Can you work these out from the model? Positions are in its coordinate system, mm. Face numbers are marked on the shaded views. A direction names the side the tool comes from. Give positions to 0.01 mm unless a question says otherwise; leave off trailing zeros. Write each loop counter-clockwise with the first axis right and the second up, starting at its lowest first coordinate (ties: lowest second). Pieces come first, ordered by that corner, then holes. Notation, with made-up numbers: (70.25, 42) -> (93.25, 42) arc R22 cw to (93.25, 62) -> close; hole circle Ø2 at (69, -35). An arc over 180 degrees is marked (long way). One line per item, written item: value.
from build123d import *

# Parameters (mm, degrees)
SKETCH1_R               = 1.5
BOSS_EXTRUDE1_DEPTH     = 1.5
SKETCH5_W               = 7.463090523
SKETCH5_H               = 8
BOSS_EXTRUDE2_DEPTH     = 3.5
CUT_EXTRUDE1_DEPTH      = 7
CUT_EXTRUDE1_DEPTH_BACK = 6
SKETCH2_W               = 2.5
SKETCH2_H               = 5.25
SKETCH3_R               = 2
CUT_EXTRUDE2_DEPTH      = 3
SKETCH6_W               = 5
SKETCH6_H               = 4
CUT_EXTRUDE3_DEPTH      = 3.5


with BuildPart() as part:
    # Sketch1 → Boss-Extrude1 (new, symmetric)
    with BuildSketch(Plane.XY):
        with BuildLine():
            Line((12, 4), (0, 4))
            ThreePointArc((0, 4), (-4, 0), (0, -4))
            Line((0, -4), (12, -4))
            Line((12, -4), (12, 4))
        make_face()
        Circle(SKETCH1_R, mode=Mode.SUBTRACT)
    extrude(amount=BOSS_EXTRUDE1_DEPTH, both=True)

    # Sketch5 → Boss-Extrude2 (add, symmetric)
    with BuildSketch(Plane.XY):
        with Locations((8.268454739, 0)):
            Rectangle(SKETCH5_W, SKETCH5_H)
    extrude(amount=BOSS_EXTRUDE2_DEPTH, both=True)

    # Sketch2 → Cut-Extrude1 (cut, two sides: drawn at the far end of the back side and taken through both)
    with BuildSketch(Plane.XY.offset(1.5).offset(-CUT_EXTRUDE1_DEPTH_BACK)):
        with Locations((8.25, 0)):
            Rectangle(SKETCH2_W, SKETCH2_H)
    extrude(amount=CUT_EXTRUDE1_DEPTH + CUT_EXTRUDE1_DEPTH_BACK, mode=Mode.SUBTRACT)

    # Sketch3 → Cut-Extrude2 (cut)
    with BuildSketch(Plane(origin=(12, 0, 0), x_dir=(0, 0, -1), z_dir=(1, 0, 0))):
        with Locations(Location((0, 0, 0), (0, 0, 90))):
            Circle(SKETCH3_R)
    extrude(amount=-CUT_EXTRUDE2_DEPTH, mode=Mode.SUBTRACT)

    # Sketch6 → Cut-Extrude3 (cut)
    with BuildSketch(Plane(origin=(0, 0, -3.5), x_dir=(-1, 0, 0), z_dir=(0, 0, -1))):
        with Locations((-12, 0)):
            Rectangle(SKETCH6_W, SKETCH6_H)
    extrude(amount=-CUT_EXTRUDE3_DEPTH, mode=Mode.SUBTRACT)


solid = part.part
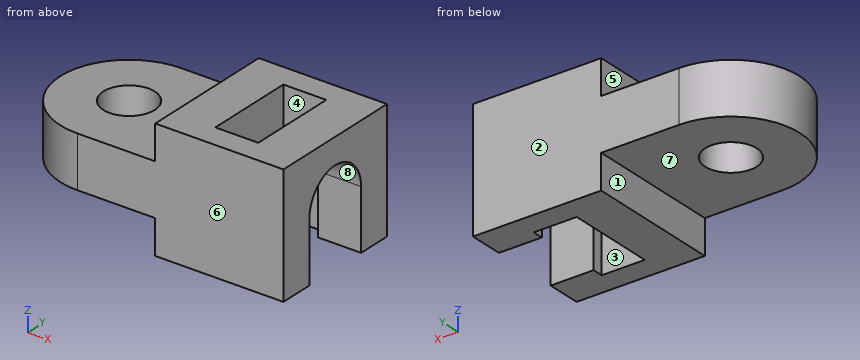
1) If we section it at C-C (x = -0.25): Write out the boundary of the cut face in (y, z).
Answer list:
outline: (-3.99, -1.5) -> (-1.48, -1.5) -> (-1.48, 1.5) -> (-3.99, 1.5) -> close; (1.48, -1.5) -> (3.99, -1.5) -> (3.99, 1.5) -> (1.48, 1.5) -> close
2) Will these pins go through, and if not, where does the flat tip stop? pin 1 (4 mm diameter, centred on x = 0, y = -0.5, fed in from +Z); pin 2 (2 mm diameter, centred on x = 3, y = -0.5, fed in from -Z); pin 3 (1.6 mm diameter, centred on y = 0.5, z = -2.5, fed in from -X).
Answer list:
pin 1: stops at z = 1.5
pin 2: stops at z = -1.5
pin 3: stops at x = 4.54
3) If we section it at D-D (z = 3.25): Write out the boundary of the cut face in (x, y) (3 decimals), and give its area (3 significant figures).
Answer list:
outline: (4.537, -4) -> (12, -4) -> (12, 4) -> (4.537, 4) -> close; hole (7, -2.625) -> (9.5, -2.625) -> (9.5, 2.625) -> (7, 2.625) -> close
area: 46.6 mm^2
4) We'd pull the mould along Y, two halves only. Please class the marked faces 1, 2 and 3: released by +Y, released by -Y, zero draft, split by the parting line, or undercut.
Answer list:
face 1: zero draft
face 2: released by +Y
face 3: undercut
5) For the marked faces 4, 5, 6, 7 and 8, which set-ups out of +Z, -Z, +X, -X, +Y, -Y let a thin tool reach every point of the face, with its end or its side?
Answer list:
face 4: +Z, -Z
face 5: +Z, -X, +Y, -Y
face 6: +Z, -Z, +X, -X, -Y
face 7: -Z, -X, +Y, -Y
face 8: -Z, +X
6) I need wall thicknesses on L1, parallel to Y at x = 0, z = 0.55; L2, parallel to X at y = 0.75, z = 2; L3, parallel to Y at x = 10.75, z = 0. Which ranges of each line are inside material? Lowest first, please.
Answer list:
L1: y = -4 to -1.5, 1.5 to 4
L2: x = 4.54 to 7, 9.5 to 12
L3: y = -4 to -2, 2 to 4
7) If we section it at A-A (y = 0): Write out the boundary of the cut face in (x, z).
Answer list:
outline: (-4, -1.5) -> (-1.5, -1.5) -> (-1.5, 1.5) -> (-4, 1.5) -> close; (1.5, -1.5) -> (4.54, -1.5) -> (4.54, -3.5) -> (7, -3.5) -> (7, 3.5) -> (4.54, 3.5) -> (4.54, 1.5) -> (1.5, 1.5) -> close; (9.5, 2) -> (12, 2) -> (12, 3.5) -> (9.5, 3.5) -> close
8) If we section it at B-B (z = -0.5): Write out the boundary of the cut face in (x, y) (3 decimals), and give its area (3 significant figures).
Answer list:
outline: (0, -4) -> (12, -4) -> (12, -2) -> (9.5, -2) -> (9.5, -2.625) -> (7, -2.625) -> (7, 2.625) -> (9.5, 2.625) -> (9.5, 2) -> (12, 2) -> (12, 4) -> (0, 4) arc R4 ccw to start; hole circle Ø3 at (0, 0)
area: 90.9 mm^2
